Answer from the drawing. Dimensions are ordinates in mm from the lowest x, y and z of the part. A direction names the side the tool comes from. Coordinates: 2 decimals unless noted, no trailing zeros. Write each loop counter-clockwise with the first axis right and the second up, starting at its lowest first coordinate (ties: lowest second). Pieces come first, ordered by that corner, then holes.
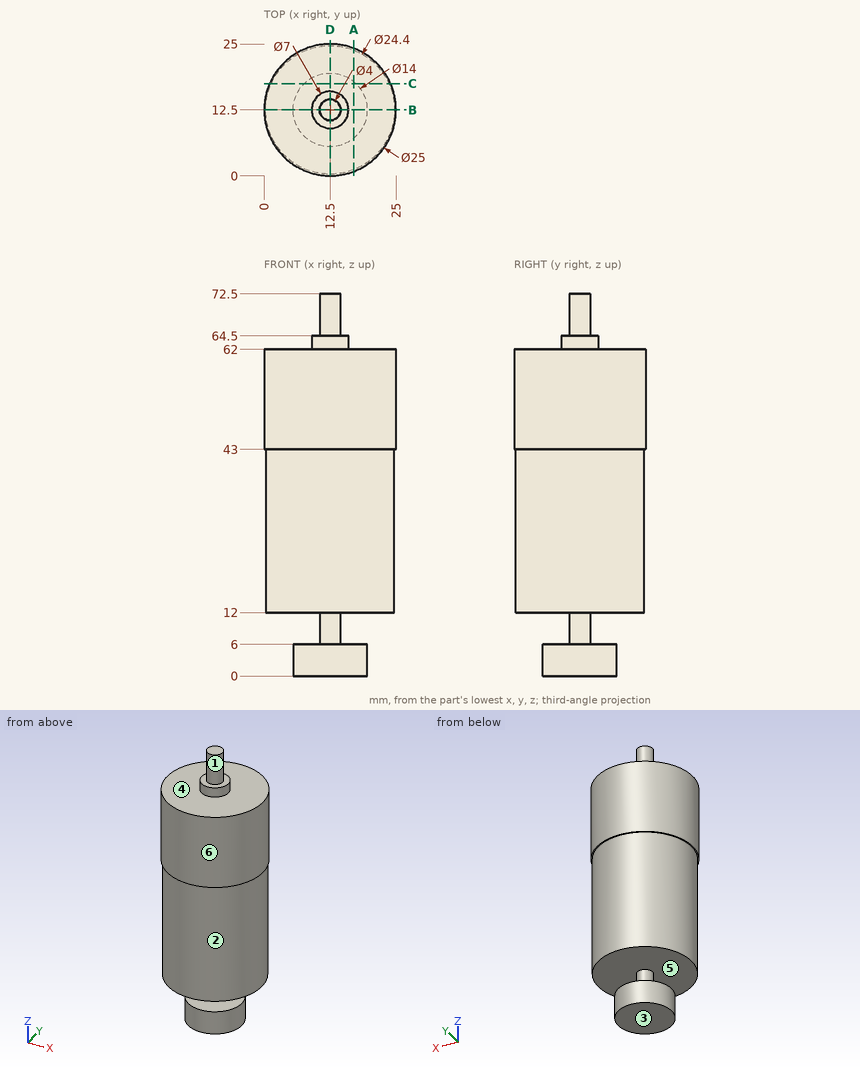
(1) Each of these flat-tipped pins is pushed along its axis until it touches: pin 1 (5 mm diameter, centred on y = 22, z = 54.5, fed in from +X); pin 2 (2 mm diameter, centred on y = 20.5, z = 10, fed in from -X); pin 3 (1.5 mm diameter, centred on y = 14.5, z = 28, fed in from -X); pin 4 (5 mm diameter, centred on x = 15, z = 33.5, fed in from -Y). Where does it stop, or does it pass through?
(2) For a pull along Z with two mould halves and no side action, classify the marked faces 3, 4, 5 and 6 as pulls with the +Z half, pulls with the -Z half, needs draft (parallel to the pull), parting line crosses it, or undercut.
(3) Find the intervals of material crossed by probe 1 along Z at (x, y) = (10.75, 7); probe 2 along Z at (x, y) = (21, 17); probe 3 along Y at (x, z) = (2.5, 39.5), in increasing order.
(4) Section C-C, the plane y = 17.5 is taken. Write down the section's boundary in (x, z), plus the area to 3 significant figures.
(5) Section A-A, the plane x = 17 is taken. Write down the section's boundary in (y, z), plus the area to 3 significant figures.
(6) Which of the six approach directions +Z, -Z, +X, -X, +Y, -Y give full straight-line access (tool end or side, diameter ignored) to the marked faces 1 and 2?
(7) Section B-B, the plane y = 12.5 is taken. Write down the section's boundary in (x, z), plus the area to 3 significant figures.
Solution:
1. pin 1: stops at x = 22.86
1. pin 2: passes through
1. pin 3: stops at x = 0.36
1. pin 4: stops at y = 0.3
2. face 3: pulls with the -Z half
2. face 4: pulls with the +Z half
2. face 5: undercut
2. face 6: needs draft
3. probe 1: z = 0 to 6, 12 to 62
3. probe 2: z = 12 to 62
3. probe 3: y = 5.51 to 19.49
4. outline: (1.04, 43) - (1.37, 43) - (1.37, 12) - (23.63, 12) - (23.63, 43) - (23.96, 43) - (23.96, 62) - (1.04, 62) - close; (7.6, 0) - (17.4, 0) - (17.4, 6) - (7.6, 6) - close
4. area: 1,180 mm2
5. outline: (0.84, 43) - (1.16, 43) - (1.16, 12) - (23.84, 12) - (23.84, 43) - (24.16, 43) - (24.16, 62) - (0.84, 62) - close; (7.14, 0) - (17.86, 0) - (17.86, 6) - (7.14, 6) - close
5. area: 1,210 mm2
6. face 1: +Z
6. face 2: -Z
7. outline: (0, 43) - (0.3, 43) - (0.3, 12) - (10.5, 12) - (10.5, 6) - (5.5, 6) - (5.5, 0) - (19.5, 0) - (19.5, 6) - (14.5, 6) - (14.5, 12) - (24.7, 12) - (24.7, 43) - (25, 43) - (25, 62) - (16, 62) - (16, 64.5) - (14.5, 64.5) - (14.5, 72.5) - (10.5, 72.5) - (10.5, 64.5) - (9, 64.5) - (9, 62) - (0, 62) - close
7. area: 1,390 mm2
